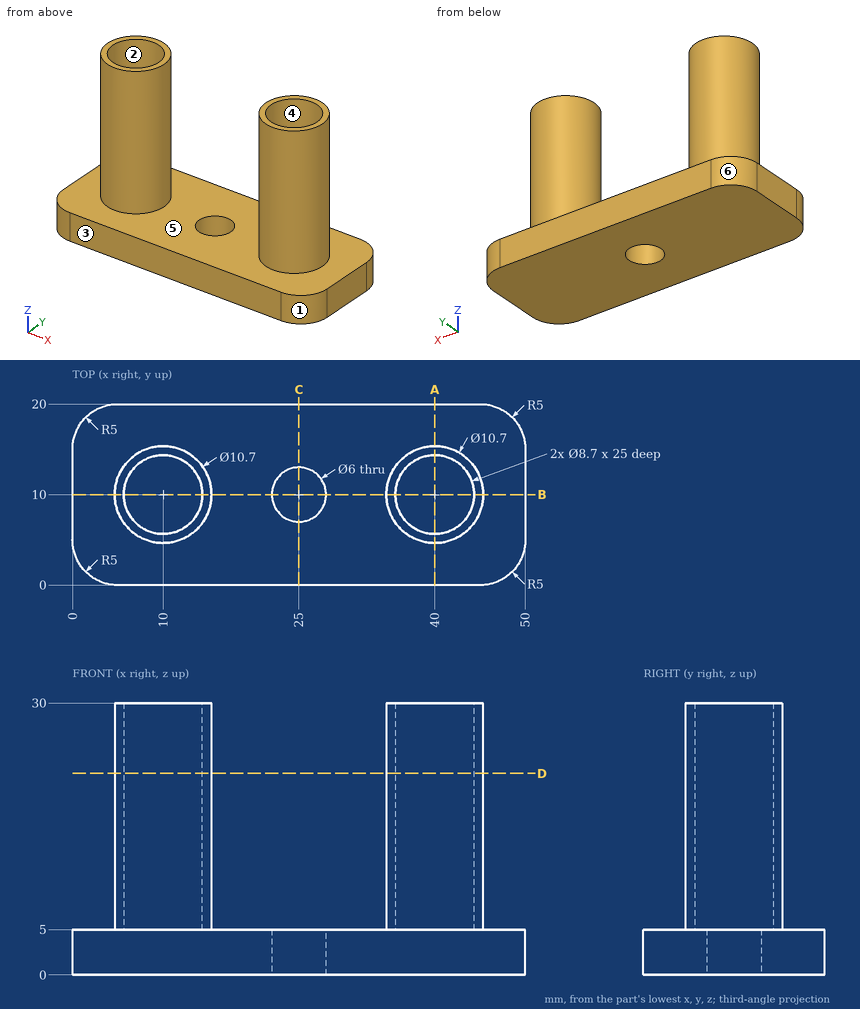
Geometry check sheet. Reference: drawing and pictorial views, mm from the part's lowest x, y, z. A direction names the side the tool comes from. Coordinates: 2 decimals unless noted, no trailing zeros. Loops run counter-clockwise (first coordinate to the right, second up) from the corner with the lowest first, then second, coordinate; pieces in that order, holes last.
1) Sectioned sample at B-B (y = 10). Record the boundary of the cut face in (x, z).
2) Access from +Z, -Z, +X, -X, +Y, -Y to the whole of each face (thin tool, end or side, straight path). Record for the marked faces 1 and 2.
3) Material ranges on probe 1 along X at (y, z) = (10, 21.5); probe 2 along X at (y, z) = (13.5, 16.5); probe 3 along Y at (x, z) = (40, 16.5), recorded low to high.
4) Sectioned sample at C-C (x = 25). Record the boundary of the cut face in (y, z), and give its area (3 significant figures).
5) Release check for a two-part mould opening along X. For the marked faces 3, 4, 5 and 6 record: released by +X, released by -X, zero draft, split by the parting line, or undercut.
6) Gauge pin test, flat ends, axial feed: pin 1 (10 mm diameter, centred on x = 25.5, y = 16.5, fed in from -Z); pin 2 (1.5 mm diameter, centred on y = 2.5, z = 3, fed in from -X); pin 3 (8 mm diameter, centred on y = 5.5, z = 18, fed in from +X); pin 4 (12 mm diameter, centred on y = 3, z = 20, fed in from -X). Record the tip position at first contact, or that the pin passes through.
7) Sectioned sample at D-D (z = 22.25). Record the boundary of the cut face in (x, y), and give its area (3 significant figures).
8) Sectioned sample at A-A (x = 40). Record the boundary of the cut face in (y, z).
Check sheet entries:
1. outline: (0, 0) - (22, 0) - (22, 5) - (15.35, 5) - (15.35, 30) - (14.35, 30) - (14.35, 5) - (5.65, 5) - (5.65, 30) - (4.65, 30) - (4.65, 5) - (0, 5) - close; (28, 0) - (50, 0) - (50, 5) - (45.35, 5) - (45.35, 30) - (44.35, 30) - (44.35, 5) - (35.65, 5) - (35.65, 30) - (34.65, 30) - (34.65, 5) - (28, 5) - close
2. face 1: +Z, -Z, +X, -Y
2. face 2: +Z
3. probe 1: x = 4.65 to 5.65, 14.35 to 15.35, 34.65 to 35.65, 44.35 to 45.35
3. probe 2: x = 5.95 to 7.42, 12.58 to 14.05, 35.95 to 37.42, 42.58 to 44.05
3. probe 3: y = 4.65 to 5.65, 14.35 to 15.35
4. outline: (0, 0) - (7, 0) - (7, 5) - (0, 5) - close; (13, 0) - (20, 0) - (20, 5) - (13, 5) - close
4. area: 70.0 mm2
5. face 3: zero draft
5. face 4: undercut
5. face 5: undercut
5. face 6: released by -X
6. pin 1: stops at z = 0
6. pin 2: stops at x = 0.32
6. pin 3: stops at x = 45.33
6. pin 4: stops at x = 4.74
7. outline: circle Ø10.7 at (10, 10); circle Ø10.7 at (40, 10); hole circle Ø8.7 at (10, 10); hole circle Ø8.7 at (40, 10)
7. area: 60.9 mm2
8. outline: (0, 0) - (20, 0) - (20, 5) - (15.35, 5) - (15.35, 30) - (14.35, 30) - (14.35, 5) - (5.65, 5) - (5.65, 30) - (4.65, 30) - (4.65, 5) - (0, 5) - close
